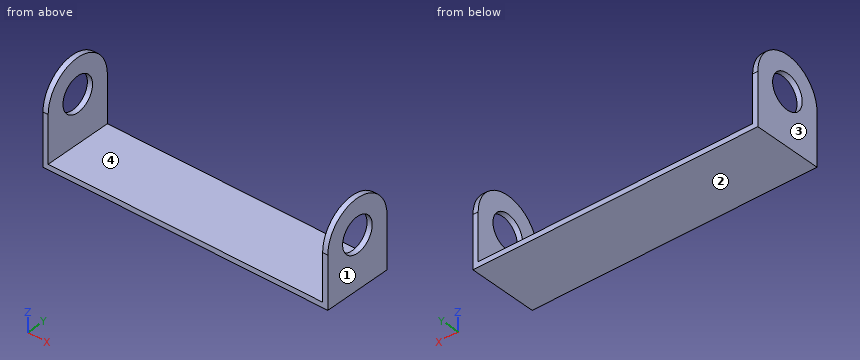
```python
from build123d import *

# Parameters (mm, degrees)
SKETCH_1_W      = 3
SKETCH_1_H      = 40
EXTRUDE_1_DEPTH = 79.5
SKETCH_2_R      = 10
EXTRUDE_2_DEPTH = 3


with BuildPart() as part:
    # 스케치1 → 보스-돌출1 (new, symmetric)
    with BuildSketch(Plane(origin=(0, 0, 0), x_dir=(0, 0, -1), z_dir=(1, 0, 0))):
        with Locations((-1.5, 0)):
            Rectangle(SKETCH_1_W, SKETCH_1_H)
    extrude(amount=EXTRUDE_1_DEPTH, both=True)

    # 스케치2 → 보스-돌출2 (add)
    with BuildSketch(Plane(origin=(79.5, 0, 0), x_dir=(0, 0, -1), z_dir=(1, 0, 0))):
        with BuildLine():
            Line((0, 20), (-30, 20))
            ThreePointArc((-30, 20), (-50, 0), (-30, -20))
            Line((-30, -20), (0, -20))
            Line((0, -20), (0, 20))
        make_face()
        with Locations((-30, 0)):
            Circle(SKETCH_2_R, mode=Mode.SUBTRACT)
    extrude_2 = extrude(amount=EXTRUDE_2_DEPTH)

    # 대칭 복사1: 보스-돌출2 across plane
    add(extrude_2.mirror(Plane(origin=(0, 0, 0), x_dir=(0, 0, 1), z_dir=(1, 0, 0))))


solid = part.part
```
For this review, take the finished solid that the model builds, in its own axes (mm). Face numbers are marked on the shaded views. Round coordinates to 2 decimals unless told otherwise and drop trailing zeros. Write each loop counter-clockwise with the first axis right and the second up, starting at its lowest first coordinate (ties: lowest second). Pieces come first, ordered by that corner, then holes.
1) Insertion check: pin 1 Ø5 at (y, z) = (-7.5, 26) entering from -X; pin 2 Ø2 at (x, y) = (-36.5, -12.5) entering from +Z. Each pin has a flat end and moves straight along its axis. Give the tip position at first contact, or say it passes through.
Answer below:
pin 1: stops at x = -82.5
pin 2: stops at z = 3
2) For line 1 along X through (y, z) = (13, 30); line 2 along Y through (x, z) = (81.6, 30); line 3 along Z through (x, y) = (-51.5, 11.5), list the stretches that pass through material, from the lowest coordinate up.
Answer below:
line 1: x = -82.5 to -79.5, 79.5 to 82.5
line 2: y = -20 to -10, 10 to 20
line 3: z = 0 to 3
3) Take a section at D-D on y = -12. Give the boundary of the cut face in (x, z).
Answer below:
outline: (-82.5, 0) - (82.5, 0) - (82.5, 46) - (79.5, 46) - (79.5, 3) - (-79.5, 3) - (-79.5, 46) - (-82.5, 46) - close
4) Mouldability with a two-part tool opening along X and no side actions: class the marked faces 1, 2, 3 and 4 as +X half, -X half, draft (parallel to the pull), parting line (faces both ways), or undercut.
Answer below:
face 1: +X half
face 2: draft
face 3: -X half
face 4: undercut
5) Take a section at C-C on y = 0. Give the boundary of the cut face in (x, z).
Answer below:
outline: (-82.5, 0) - (82.5, 0) - (82.5, 20) - (79.5, 20) - (79.5, 3) - (-79.5, 3) - (-79.5, 20) - (-82.5, 20) - close; (-82.5, 40) - (-79.5, 40) - (-79.5, 50) - (-82.5, 50) - close; (79.5, 40) - (82.5, 40) - (82.5, 50) - (79.5, 50) - close
6) Take a section at B-B on z = 11.5. Give the boundary of the cut face in (x, y).
Answer below:
outline: (-82.5, -20) - (-79.5, -20) - (-79.5, 20) - (-82.5, 20) - close; (79.5, -20) - (82.5, -20) - (82.5, 20) - (79.5, 20) - close
7) Take a section at A-A on z = 24. Give the boundary of the cut face in (x, y), then the cut area to 3 significant figures.
Answer below:
outline: (-82.5, -20) - (-79.5, -20) - (-79.5, -8) - (-82.5, -8) - close; (-82.5, 8) - (-79.5, 8) - (-79.5, 20) - (-82.5, 20) - close; (79.5, -20) - (82.5, -20) - (82.5, -8) - (79.5, -8) - close; (79.5, 8) - (82.5, 8) - (82.5, 20) - (79.5, 20) - close
area: 144 mm2
